Work out the finished part from the listing and answer in its coordinate system (mm). A direction names the side the tool comes from. Round coordinates to 2 decimals unless told otherwise and drop trailing zeros. Write each loop counter-clockwise with the first axis right and the second up, starting at its lowest first coordinate (ties: lowest second). Pieces come first, ordered by that corner, then holes. Notation, with made-up numbers: (86.25, -29.75) - (108.25, -29.75) arc R30 cw to (108.25, -1.75) - close; hole circle Ø10 at (73.25, -1.5). An arc over 180 degrees is marked (long way). Answer as a JSON object with one key per item and string values.
```python
from build123d import *

# Parameters (mm, degrees)
BOSS_EXTRUDE2_DEPTH = 12.7
BOSS_EXTRUDE3_DEPTH = 43.18
BOSS_EXTRUDE4_DEPTH = 8.89
SKETCH10_R          = 9.398
CUT_EXTRUDE2_DEPTH  = 9.398
FILLET1_R           = 0.508
SKETCH11_R          = 1.397
CUT_EXTRUDE3_DEPTH  = 0.254
SKETCH12_R          = 3.81
CUT_EXTRUDE5_DEPTH  = 2.54
CUT_EXTRUDE6_REACH  = 31.845


with BuildPart() as part:
    # Sketch2 → Revolve1 (revolve)
    with BuildSketch(Plane(origin=(0, 0, 0), x_dir=(0, 0, -1), z_dir=(1, 0, 0))):
        with BuildLine():
            Line((0, 18.923), (4.318, 16.764))
            Line((4.318, 16.764), (18.542, 16.764))
            ThreePointArc((18.542, 16.764), (18.721605122, 16.689605122), (18.796, 16.51))
            Line((18.796, 16.51), (18.796, 9.398))
            Line((18.796, 9.398), (17.78, 9.398))
            Line((17.78, 9.398), (17.78, 9.652))
            Line((17.78, 9.652), (18.542, 9.652))
            Line((18.542, 9.652), (18.542, 16.256))
            ThreePointArc((18.542, 16.256), (18.467605122, 16.435605122), (18.288, 16.51))
            Line((18.288, 16.51), (4.258038734, 16.51))
            Line((4.258038734, 16.51), (0, 18.639019367))
            Line((0, 18.639019367), (0, 18.923))
        make_face()
    revolve(axis=Axis((0, 0, 8.948655539), (0, 0, -1)))



with BuildPart() as body_2:
    # Sketch6 → Boss-Extrude2 (new body)
    with BuildSketch(Plane(origin=(16.764, 0, 0), x_dir=(0, 0, -1), z_dir=(1, 0, 0))):
        with BuildLine():
            Line((26.924, 19.558), (27.178, 19.558))
            Line((27.178, 19.558), (27.178, 12.92200108))
            ThreePointArc((27.178, 12.92200108), (26.517818368, 11.328181632), (24.92399892, 10.668))
            Line((24.92399892, 10.668), (19.05, 10.668))
            Line((19.05, 10.668), (19.05, -10.668))
            Line((19.05, -10.668), (24.92399892, -10.668))
            ThreePointArc((24.92399892, -10.668), (26.517818368, -11.328181632), (27.178, -12.92200108))
            Line((27.178, -12.92200108), (27.178, -15.24))
            Line((27.178, -15.24), (26.924, -15.24))
            Line((26.924, -15.24), (26.924, -12.92200108))
            ThreePointArc((26.924, -12.92200108), (26.338213246, -11.507786754), (24.92399892, -10.922))
            Line((24.92399892, -10.922), (18.796, -10.922))
            Line((18.796, -10.922), (18.796, 10.922))
            Line((18.796, 10.922), (24.92399892, 10.922))
            ThreePointArc((24.92399892, 10.922), (26.338213246, 11.507786754), (26.924, 12.92200108))
            Line((26.924, 12.92200108), (26.924, 19.558))
        make_face()
    extrude(amount=BOSS_EXTRUDE2_DEPTH)


with BuildPart() as part_1:
    add(part.part)

    add(body_2.part)  # Boss-Extrude3 merges body 2
    # Sketch8 → Boss-Extrude3 (add)
    with BuildSketch(Plane.ZY.offset(-16.764)):
        with BuildLine():
            Line((-26.924, 12.92200108), (-26.924, 19.558))
            Line((-26.924, 19.558), (-27.178, 19.558))
            Line((-27.178, 19.558), (-27.178, 12.92200108))
            ThreePointArc((-27.178, 12.92200108), (-26.517818368, 11.328181632), (-24.92399892, 10.668))
            Line((-24.92399892, 10.668), (-19.05, 10.668))
            Line((-19.05, 10.668), (-19.05, -10.668))
            Line((-19.05, -10.668), (-24.92399892, -10.668))
            ThreePointArc((-24.92399892, -10.668), (-26.517818368, -11.328181632), (-27.178, -12.92200108))
            Line((-27.178, -12.92200108), (-27.178, -15.24))
            Line((-27.178, -15.24), (-26.924, -15.24))
            Line((-26.924, -15.24), (-26.924, -12.92200108))
            ThreePointArc((-26.924, -12.92200108), (-26.338213246, -11.507786754), (-24.92399892, -10.922))
            Line((-24.92399892, -10.922), (-18.796, -10.922))
            Line((-18.796, -10.922), (-18.796, 10.922))
            Line((-18.796, 10.922), (-24.92399892, 10.922))
            ThreePointArc((-24.92399892, 10.922), (-26.338213246, 11.507786754), (-26.924, 12.92200108))
        make_face()
    extrude(amount=BOSS_EXTRUDE3_DEPTH)

    # Sketch9 → Boss-Extrude4 (add)
    with BuildSketch(Plane.ZY.offset(26.416)):
        with BuildLine():
            Line((-18.796, 11.58899892), (-18.796, -11.58899892))
            ThreePointArc((-18.796, -11.58899892), (-19.381786754, -13.003213246), (-20.79600108, -13.589))
            Line((-20.79600108, -13.589), (-26.67, -13.589))
            Line((-26.67, -13.589), (-26.67, -13.335))
            Line((-26.67, -13.335), (-20.79600108, -13.335))
            ThreePointArc((-20.79600108, -13.335), (-19.561391876, -12.823608124), (-19.05, -11.58899892))
            Line((-19.05, -11.58899892), (-19.05, 11.58899892))
            ThreePointArc((-19.05, 11.58899892), (-19.599773222, 12.827111013), (-20.855647788, 13.335))
            Line((-20.855647788, 13.335), (-26.67, 13.335))
            Line((-26.67, 13.335), (-26.67, 13.589))
            Line((-26.67, 13.589), (-20.79600108, 13.589))
            ThreePointArc((-20.79600108, 13.589), (-19.381786754, 13.003213246), (-18.796, 11.58899892))
        make_face()
    extrude(amount=BOSS_EXTRUDE4_DEPTH)

    # Sketch10 → Cut-Extrude2 (cut)
    with BuildSketch(Plane.XY.offset(-18.796)):
        Circle(SKETCH10_R)
    extrude(amount=-CUT_EXTRUDE2_DEPTH, mode=Mode.SUBTRACT)

    # Fillet1
    fillet1_edges = [part_1.edges().sort_by_distance(p)[0] for p in [
        (-9.398, 0, -19.05),
    ]]
    fillet(fillet1_edges, radius=FILLET1_R)

    # Sketch11 → Cut-Extrude3 (cut)
    with BuildSketch(Plane(origin=(0, 0, -27.178), x_dir=(-1, 0, 0), z_dir=(0, 0, -1))):
        with Locations((6.35, 14.351)):
            Circle(SKETCH11_R)
    extrude(amount=-CUT_EXTRUDE3_DEPTH, mode=Mode.SUBTRACT)

    # Sketch12 → Cut-Extrude5 (cut)
    with BuildSketch(Plane(origin=(0, 0, -27.178), x_dir=(-1, 0, 0), z_dir=(0, 0, -1))):
        with Locations((16.764, 21.463)):
            Circle(SKETCH12_R)
        with Locations((-4.064, 21.463)):
            Circle(SKETCH12_R)
    extrude(amount=-CUT_EXTRUDE5_DEPTH, mode=Mode.SUBTRACT)

    # Sketch13 → Cut-Extrude6 (cut, up to next)
    with BuildSketch(Plane(origin=(0, 10.922, 0), x_dir=(1, 0, 0), z_dir=(0, 1, 0)), mode=Mode.PRIVATE) as cut_extrude6_sk1:
        with BuildLine():
            Line((4.318, 24.309866454), (8.382, 24.309866454))
            ThreePointArc((8.382, 24.309866454), (8.561605122, 24.235471576), (8.636, 24.055866454))
            Line((8.636, 24.055866454), (8.636, 19.991866454))
            ThreePointArc((8.636, 19.991866454), (8.561605122, 19.812261332), (8.382, 19.737866454))
            Line((8.382, 19.737866454), (4.318, 19.737866454))
            ThreePointArc((4.318, 19.737866454), (4.138394878, 19.812261332), (4.064, 19.991866454))
            Line((4.064, 19.991866454), (4.064, 24.055866454))
            ThreePointArc((4.064, 24.055866454), (4.138394878, 24.235471576), (4.318, 24.309866454))
        make_face()
    cut_extrude6_tool1 = extrude(cut_extrude6_sk1.sketch, amount=-CUT_EXTRUDE6_REACH, mode=Mode.PRIVATE) & part_1.part
    add(cut_extrude6_tool1.solids().sort_by_distance((6.35, 10.922, -22.023866))[0], mode=Mode.SUBTRACT)


solid = part_1.part
```
Item 1: Determine the mould class of faces 1 (the flat face through (2, -10.922, -22)), 2 (the conical face through (5.07, 16.09, -4.11)), 3 (the cylindrical face through (-5.87, -7.66, -18.17)) for opening direction X: pulls with the +X half, pulls with the -X half, needs draft (parallel to the pull), parting line crosses it, or undercut.
Results found:
{"face 1": "needs draft", "face 2": "parting line crosses it", "face 3": "undercut"}
Item 2: A cutting plane is placed at B-B (x = 21.5). Write down the section's boundary in (y, z).
Results found:
{"outline": "(-15.24, -27.18) - (-12.92, -27.18) arc R2.25 ccw to (-10.67, -24.92) - (-10.67, -19.05) - (10.67, -19.05) - (10.67, -24.92) arc R2.25 ccw to (12.92, -27.18) - (19.56, -27.18) - (19.56, -26.92) - (12.92, -26.92) arc R2 cw to (10.92, -24.92) - (10.92, -18.8) - (-10.92, -18.8) - (-10.92, -24.92) arc R2 cw to (-12.92, -26.92) - (-15.24, -26.92) - close"}
Item 3: For faces 4 (the cylindrical face through (1.92, 11.35, -26.54)), 5 (the flat face through (2, 16, -27.178)), 6 (the cylindrical face through (1.92, -11.52, -26.35)), 7 (the flat face through (0, 13, -18.796)), 8 (the flat face through (-7, -7, -18.542)), determine the directions among +Z, -Z, +X, -X, +Y, -Y from which every point of the face is accessible in a straight line to the end or side of a thin tool.
Results found:
{"face 4": "-Z, +X, -X", "face 5": "-Z, +X, -X, +Y, -Y", "face 6": "+X, -X, -Y", "face 7": "+X, +Y", "face 8": "+Z"}
Item 4: Consider line 1 along X through (y, z) = (0, -17.95); line 2 along Y through (x, z) = (22, -25); line 3 along Z through (x, y) = (6, -8). Determine where each line is inside the solid, lowest interval first.
Results found:
{"line 1": "-16.76 to -16.51, -9.65 to -9.4, 9.4 to 9.65, 16.51 to 16.76", "line 2": "-10.92 to -10.67, 10.67 to 10.92", "line 3": "-19.05 to -18.54"}
Item 5: A cutting plane is placed at D-D (x = 5.5). Give the number of separate pieces and of enclosed holes in the cut face, and give its area (3 significant figures).
Results found:
{"separate pieces": "3", "enclosed holes": "0", "area": "21.8 mm²"}
Item 6: Each of these flat-tipped pins is pushed along its axis until it touches: P1, Ø1.8, axis at x = 1.5, z = -21.5, coming from the -Y side; P2, Ø10, axis at x = 16.5, z = -16, coming from the -Y side; P3, Ø4, axis at y = -14, z = -11, coming from the -X side. Where does it stop, or does it pass through?
Results found:
{"P1": "y = -10.92", "P2": "y = -12.2", "P3": "x = -11.71"}
Item 7: A cutting plane is placed at C-C (z = -12.25). Write down the section's boundary in (x, y).
Results found:
{"outline": "circle Ø33.53 at (0, 0); hole circle Ø33.02 at (0, 0)"}
